from build123d import *

# Parameters (mm, degrees)
F1_DEPTH = 24.8
F2_R     = 0.2


with BuildPart() as f1:
    # F0 (on Front) → F1 (new body)
    with BuildSketch(Plane.XZ):
        Polygon((10.026696, 9.973304), (0, 20), (0, 14.152517), (-14.131747, 14.152517), (-9.989615, 10.010385), (-20, 0), (-14.115414, 0), (-14.115414, -14.168807), (-9.973304, -10.026696), (0, -20), (0, -14.131747), (14.152517, -14.131747), (10.010385, -9.989615), (20, 0), (14.168807, 0), (14.168807, 14.115414), align=None)
        with BuildLine():
            ThreePointArc((0, -2.5), (-1.767767, 1.767767), (2.5, 0))
            ThreePointArc((2.5, 0), (1.767767, -1.767767), (0, -2.5))
        make_face(mode=Mode.SUBTRACT)
    extrude(amount=F1_DEPTH)

    # F2
    f2_edges = [f1.edges().sort_by_distance(p)[0] for p in [
        (0, -12.4, 20),
        (14.168807, -12.4, 14.115414),
        (20, -12.4, 0),
        (14.152517, -12.4, -14.131747),
        (0, -12.4, -20),
        (-12.044359, -24.8, -12.097752),
        (-20, -12.4, 0),
        (-14.131747, -12.4, 14.152517),
    ]]
    fillet(f2_edges, radius=F2_R)


solid = f1.part
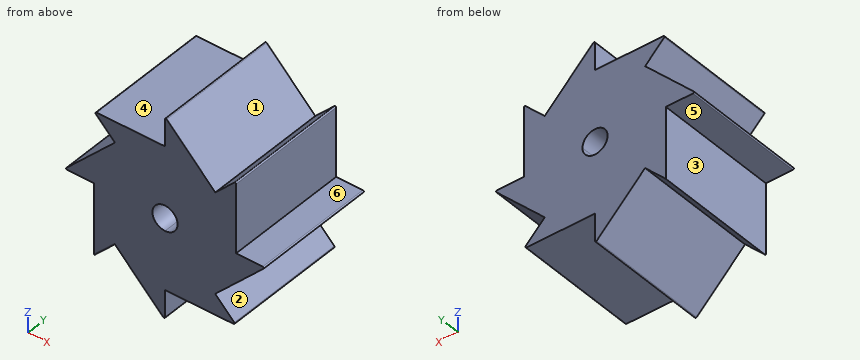
Input: part model. Units: mm. Frame: model coordinates. Face numbers are marked on the shaded views. A direction names the side the tool comes from. Give positions to 0.01 mm unless a question says otherwise; leave off trailing zeros. Write each loop counter-clockwise with the first axis right and the second up, starting at its lowest first coordinate (ties: lowest second). Pieces come first, ordered by that corner, then holes. Notation, with made-up numbers: M 1,45.25 L 20,45.25 A27 cw 20,67.25 Z; hole C 44,6 d7. An arc over 180 degrees is marked long. Use one line per item in the form item = value.
1. Cut plane A-A on y = -21.5. Return loops of the section in (x, z).
Outcome:
outline = M -19.66,0.34 A0.2 ccw -19.52,0 L -14.12,0 L -14.12,-14.17 L -9.97,-10.03 L -0.34,-19.66 A0.2 ccw 0,-19.52 L 0,-14.13 L 13.67,-14.13 A0.2 ccw 13.81,-13.79 L 10.01,-9.99 L 19.66,-0.34 A0.2 ccw 19.52,0 L 14.17,0 L 14.17,13.63 A0.2 ccw 13.83,13.77 L 10.03,9.97 L 0.34,19.66 A0.2 ccw 0,19.52 L 0,14.15 L -13.65,14.15 A0.2 ccw -13.79,13.81 L -9.99,10.01 Z; hole C 0,0 d5
2. First-contact query: P1, Ø4, axis at y = -18.5, z = 5.5, coming from the +X side; P2, Ø1.6, axis at x = 17, y = -7.5, coming from the +Z side; P3, Ø4, axis at x = 7, y = -12.5, coming from the -Z side. Flat tips, straight axial feed; report the tip coordinate or a pass-through.
Outcome:
P1 = 14.17
P2 = 0
P3 = -14.13
3. Cut plane D-D on x = 16. Return loops of the section in (y, z), and give its area (3 significant figures).
Outcome:
outline = M -24.8,-4 L 0,-4 L 0,0 L -24.8,0 Z
area = 99.2 mm²
4. Cut plane B-B on z = -1.5. Return loops of the section in (x, y), and give its area (3 significant figures).
Outcome:
outline = M -14.12,-24.8 L -2,-24.8 L -2,0 L -14.12,0 Z; M 2,-24.8 L 18.5,-24.8 L 18.5,0 L 2,0 Z
area = 710 mm²
5. Cut plane C-C on x = 1. Return loops of the section in (y, z).
Outcome:
outline = M -24.8,-14.13 L 0,-14.13 L 0,-2.29 L -24.8,-2.29 Z; M -24.8,2.29 L 0,2.29 L 0,19 L -24.8,19 Z
6. Mould query, pull axis X, two halves, no side actions, for the marked faces 1, 2 and 3. Classes: released by +X, released by -X, zero draft, split by the parting line, or undercut.
Outcome:
face_1 = undercut
face_2 = released by +X
face_3 = released by -X
7. Ray query, L1, parallel to Z at x = -2, y = -8.5; L2, parallel to X at y = -3.75, z = 1.5; L3, parallel to Z at x = 12, y = -5.5. Return the intervals inside material, ascending.
Outcome:
L1 = -18 to -1.5, 1.5 to 14.15
L2 = -18.5 to -2, 2 to 14.17
L3 = -14.13 to -11.98, -8 to 11.95
8. Reachability of the marked faces 4, 5 and 6 from +Z, -Z, +X, -X, +Y, -Y: full face, straight path, thin tool, end or side. Return the list, or none.
Outcome:
face_4 = +Z, -X, +Y, -Y
face_5 = -Z, -X, +Y, -Y
face_6 = +Z, +X, +Y, -Y
